The model under review builds one solid part; all positions refer to its coordinate system, in mm. A direction names the side the tool comes from. Give positions to 0.01 mm unless a question says otherwise; leave off trailing zeros. Loops run counter-clockwise (first coordinate to the right, second up) from the corner with the lowest first, then second, coordinate; pieces in that order, holes last. Notation, with made-up numbers: M 72.5,13.5 L 77.5,13.5 A15 cw 77.5,31.5 Z; hole C 33,54 d5. An arc over 180 degrees is marked long. One line per item, written item: value. Start each with the question number.
Q1. Mouldability with a two-part tool opening along X and no side actions: class faces 4 (the face through (-22.36, 5.19, 21.1)), 5 (the face through (-43.61, -24.01, 0.99)), 6 (the face through (47.5, 0, 1)), 7 (the face through (-1, -28, 1)) as released by +X, released by -X, zero draft, split by the parting line, or undercut.
Q2. We need section A-A on x = -42.5. Write out the cut boundary in (y, z), plus the area to 3 significant figures.
Q3. We need section C-C on z = 17.75. Write out the cut boundary in (x, y).
Q4. We need section D-D on x = -12. Write out the cut boundary in (y, z), plus the area to 3 significant figures.
Q5. For faces 1 (the face through (-8, -2.7, 10)), 2 (the face through (-15.36, -15.33, 21.1)), 3 (the face through (40.5, -15, 10)), list the 3-axis set-ups (+Z, -Z, +X, -X, +Y, -Y) from which the entire face can be reached by the end or side of a thin tool; tool diameter is ignored.
Q6. For pin 1 (13 mm diameter, centred on y = 3, z = 10.5, fed in from +X); pin 2 (10 mm diameter, centred on x = 16.5, y = 7, fed in from +Z); pin 3 (13 mm diameter, centred on y = 7.5, z = 10, fed in from -X), all flat-tipped, find the tip position at first contact; note any pin that passes through.
Q7. To check wall thickness, follow line 1 along Y through (x, z) = (-42.5, 1.05); line 2 along X through (y, z) = (-14.5, 11.25); line 3 along X through (y, z) = (-18, 21.25). State the ranges of each line that lie inside material, in increasing order. Write a range as from..to.
Q8. We need section B-B on y = 23. Write out the cut boundary in (x, z), plus the area to 3 significant figures.
Solid Edge part; units mm, degrees
sketch "Sketch1" plane through (0, 0, 0) normal (0, 0, 1) x (1, 0, 0)
  line L0 (-47.5, 28) -> (-47.5, -28)
  line L1 (-47.5, -28) -> (47.5, -28)
  line L2 (47.5, -28) -> (47.5, 28)
  line L3 (47.5, 28) -> (-47.5, 28)
  circle A0 centre (-42.5, 23) radius 1.5
  circle A1 centre (-42.5, -23) radius 1.5
  circle A2 centre (43.5, -23) radius 1.5
  circle A3 centre (43.5, 23) radius 1.5
extrude "Protrusion1" add sketch "Sketch1" along normal blind 2
sketch "Sketch2" plane through (0, 0, 0) normal (0, 0, -1) x (1, 0, 0)
  line L0 (-21.5, -13.3) -> (-21.5, 2.7)
  line L1 (-21.5, 2.7) -> (-38.5, 2.7)
  line L2 (-38.5, 2.7) -> (-38.5, -13.3)
  line L3 (-38.5, -13.3) -> (-21.5, -13.3)
  line L4 (-16.218, 2.7) -> (-16.218, -13.3)
  line L5 (-16.218, -13.3) -> (0.782, -13.3)
  line L6 (0.782, -13.3) -> (0.782, 2.7)
  line L7 (0.782, 2.7) -> (-16.218, 2.7)
  line L8 (3.6956, 23.4371) -> (3.6956, 7.4371)
  line L9 (3.6956, 7.4371) -> (20.6956, 7.4371)
  line L10 (20.6956, 7.4371) -> (20.6956, 23.4371)
  line L11 (20.6956, 23.4371) -> (3.6956, 23.4371)
  line L12 (23.5, 23.4371) -> (23.5, 7.4371)
  line L13 (23.5, 7.4371) -> (40.5, 7.4371)
  line L14 (40.5, 7.4371) -> (40.5, 23.4371)
  line L15 (40.5, 23.4371) -> (23.5, 23.4371)
  line L16 (-38.5375, 23.4371) -> (-38.5375, 7.4371)
  line L17 (-38.5375, 7.4371) -> (-21.5375, 7.4371)
  line L18 (-21.5375, 7.4371) -> (-21.5375, 23.4371)
  line L19 (-21.5375, 23.4371) -> (-38.5375, 23.4371)
  line L20 (-16.218, 23.4371) -> (-16.218, 7.4371)
  line L21 (-16.218, 7.4371) -> (0.782, 7.4371)
  line L22 (0.782, 7.4371) -> (0.782, 23.4371)
  line L23 (0.782, 23.4371) -> (-16.218, 23.4371)
extrude "ExtrudedProtrusion_2" add sketch "Sketch2" against normal blind 22
fillet "Round_1" radius 3 24 edges at (-38.5, 5.3, 22) (-30, -2.7, 22) (-21.5, 5.3, 22) (-16.218, 5.3, 22) (-30, 13.3, 22) (-7.718, -2.7, 22) (0.782, 5.3, 22) (-7.718, 13.3, 22) (-38.5375, -15.4371, 22) (-30.0375, -23.4371, 22) (-21.5375, -15.4371, 22) (-30.0375, -7.4371, 22) (-16.218, -15.4371, 22) (-7.718, -7.4371, 22) (-7.718, -23.4371, 22) (0.782, -15.4371, 22) (3.6956, -15.4371, 22) (12.1956, -23.4371, 22) (12.1956, -7.4371, 22) (20.6956, -15.4371, 22) (23.5, -15.4371, 22) (32, -23.4371, 22) (40.5, -15.4371, 22) (32, -7.4371, 22)
Solved:
1. face 4: undercut
1. face 5: undercut
1. face 6: released by +X
1. face 7: zero draft
2. outline: M -28,0 L -24.5,0 L -24.5,2 L -28,2 Z; M -21.5,0 L 21.5,0 L 21.5,2 L -21.5,2 Z; M 24.5,0 L 28,0 L 28,2 L 24.5,2 Z
2. area: 100 mm2
3. outline: M -38.54,-23.44 L -21.54,-23.44 L -21.54,-7.44 L -38.54,-7.44 Z; M -38.5,-2.7 L -21.5,-2.7 L -21.5,13.3 L -38.5,13.3 Z; M -16.22,-23.44 L 0.78,-23.44 L 0.78,-7.44 L -16.22,-7.44 Z; M -16.22,-2.7 L 0.78,-2.7 L 0.78,13.3 L -16.22,13.3 Z; M 3.7,-23.44 L 20.7,-23.44 L 20.7,-7.44 L 3.7,-7.44 Z; M 23.5,-23.44 L 40.5,-23.44 L 40.5,-7.44 L 23.5,-7.44 Z
4. outline: M -28,0 L 28,0 L 28,2 L 13.3,2 L 13.3,19 A3 ccw 10.3,22 L 0.3,22 A3 ccw -2.7,19 L -2.7,2 L -7.44,2 L -7.44,19 A3 ccw -10.44,22 L -20.44,22 A3 ccw -23.44,19 L -23.44,2 L -28,2 Z
4. area: 744 mm2
5. face 1: +Z, +X, -X
5. face 2: +Z, +Y, -Y
5. face 3: +Z, +X, +Y, -Y
6. pin 1: x = 0.78
6. pin 2: z = 2
6. pin 3: x = -38.5
7. line 1: -28..-24.5, -21.5..21.5, 24.5..28
7. line 2: -38.54..-21.54, -16.22..0.78, 3.7..20.7, 23.5..40.5
7. line 3: -37.52..-22.55, -15.2..-0.23, 4.71..19.68, 24.52..39.48
8. outline: M -47.5,0 L -44,0 L -44,2 L -47.5,2 Z; M -41,0 L 42,0 L 42,2 L -41,2 Z; M 45,0 L 47.5,0 L 47.5,2 L 45,2 Z
8. area: 178 mm2
